```python
from build123d import *

# Parameters (mm, degrees)
F1_DEPTH = 25.4
F2_R     = 10
F3_DEPTH = 25.4


with BuildPart() as f1:
    # F0 (on Top) → F1 (new body)
    with BuildSketch(Plane.XY):
        with BuildLine():
            Line((50, 50), (-35, 50))
            ThreePointArc((-35, 50), (-45.606602, 45.606602), (-50, 35))
            Line((-50, 35), (-50, -50))
            Line((-50, -50), (35, -50))
            ThreePointArc((35, -50), (45.606602, -45.606602), (50, -35))
            Line((50, -35), (50, 50))
        make_face()
    extrude(amount=F1_DEPTH)

    # F2 (on face) → F3 (cut, through all)
    with BuildSketch(Plane.XY.offset(25.4)):
        with Locations((-25, 25)):
            Circle(F2_R)
        with Locations((25, -25)):
            Circle(F2_R)
    extrude(amount=-F3_DEPTH, mode=Mode.SUBTRACT)


solid = f1.part
```
Geometry: final body of the model. Coordinates: model frame, mm. Give positions to 0.01 mm unless a question says otherwise; leave off trailing zeros. Order: outer loops, then holes, each group sorted by start corner. A loop starts at its lowest first (then second) coordinate and runs counter-clockwise, first axis right, second up. Notation, with made-up numbers: M 12,70 L 30,70 A22 ccw 30,88 Z; hole C 0.5,19 d8. An arc over 180 degrees is marked long. Answer as CSV lines item,"result". Start each with the question number.
1) Mould query, pull axis X, two halves, no side actions, for faces 1 (the flat face through (-50, -7, 13)), 2 (the flat face through (-1, 1, 0)), 3 (the cylindrical face through (34.54, -22, 12.88)). Classes: +X half, -X half, draft (parallel to the pull), parting line (faces both ways), or undercut.
2) First-contact query: P1, Ø18, axis at x = -25, y = 25, coming from the +Z side. Flat tip, straight axial feed; report the tip coordinate or a pass-through.
3) Cut plane D-D (y = -43). Output: boundary loops of the cut face in (x, z), then the cut area to 3 significant figures.
4) Cut plane A-A (y = 25). Output: boundary loops of the cut face in (x, z), then the cut area to 3 significant figures.
5) Line query: line 1 (Y direction, x = -25.5, z = 5); line 2 (Y direction, x = 25, z = 9); line 3 (X direction, y = 35.5, z = 6). Output: solid intervals per line, ascending. Write a range as from..to.
6) Cut plane B-B (x = -25). Output: boundary loops of the cut face in (y, z).
7) Cut plane C-C (z = 9.25). Output: boundary loops of the cut face in (x, y).
Findings below:
1,face 1,"-X half"
1,face 2,"draft"
1,face 3,"undercut"
2,P1,"passes through"
3,outline,"M -50,0 L 47.69,0 L 47.69,25.4 L -50,25.4 Z"
3,area,"2,480 mm²"
4,outline,"M -50,0 L -35,0 L -35,25.4 L -50,25.4 Z; M -15,0 L 50,0 L 50,25.4 L -15,25.4 Z"
4,area,"2,030 mm²"
5,line 1,"y = -50..15.01, 34.99..50"
5,line 2,"y = -50..-35, -15..50"
5,line 3,"x = -49.99..50"
6,outline,"M -50,0 L 15,0 L 15,25.4 L -50,25.4 Z; M 35,0 L 50,0 L 50,25.4 L 35,25.4 Z"
7,outline,"M -50,-50 L 35,-50 A15 ccw 50,-35 L 50,50 L -35,50 A15 ccw -50,35 Z; hole C -25,25 d20; hole C 25,-25 d20"
